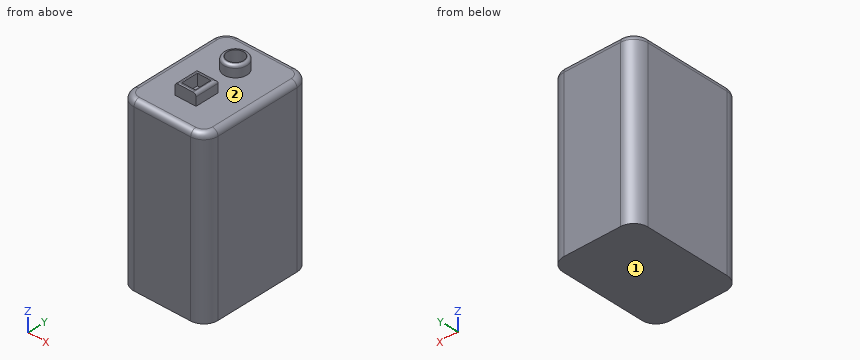
Autodesk Inventor part; units mm, degrees
ref_plane "YZ Plane" through (0, 0, 0) normal (1, 0, 0) x (0, 1, 0)
ref_plane "XZ Plane" through (0, 0, 0) normal (0, 1, 0) x (-1, 0, 0)
ref_plane "XY Plane" through (0, 0, 0) normal (0, 0, 1) x (1, 0, 0)
sketch "Sketch1" plane through (0, 0, 0) normal (1, 0, 0) x (0, 1, 0)
  line L0 (43.6864, 61.8662) -> (-7.1136, 61.8662)
  line L1 (-7.1136, 61.8662) -> (-7.1136, -14.3338)
  line L2 (-7.1136, -14.3338) -> (43.6864, -14.3338)
  line L3 (43.6864, -14.3338) -> (43.6864, 61.8662)
  point P0 (0, 0)
extrude "Extrusion1" add sketch "Sketch1" along normal blind 38.1
fillet "Fillet1" radius 6.35 4 edges at (38.1, 43.6864, 23.7662) (0, 43.6864, 23.7662) (38.1, -7.1136, 23.7662) (0, -7.1136, 23.7662)
sketch "Sketch2" plane through (0, -0.7636, 61.8662) normal (0, 0, 1) x (1, 0, 0)
  circle A0 centre (18.3636, 29.6461) radius 5.1979
  line L0 (14.0847, 15.7397) -> (23.5615, 15.7397)
  line L1 (23.5615, 15.7397) -> (23.5615, 5.0424)
  line L2 (23.5615, 5.0424) -> (14.0847, 5.0424)
  line L3 (14.0847, 5.0424) -> (14.0847, 15.7397)
  point P0 (0, 0.7636)
extrude "Extrusion2" add sketch "Sketch2" along normal blind 5.08
sketch "Sketch3" plane through (18.3636, 28.8825, 66.9462) normal (0, 0, 1) x (1, 0, 0)
  circle A0 centre (0, 0) radius 3.6755
  point P0 (-18.3636, -28.8825)
extrude "Extrusion3" cut sketch "Sketch3" against normal blind 5.08
sketch "Sketch4" plane through (0, -0.7636, 66.9462) normal (0, 0, 1) x (1, 0, 0)
  line L0 (15.8676, 13.9568) -> (21.9293, 13.9568)
  line L1 (21.9293, 13.9568) -> (21.9293, 7.1819)
  line L2 (21.9293, 7.1819) -> (15.8676, 7.1819)
  line L3 (15.8676, 7.1819) -> (15.8676, 13.9568)
  point P0 (0, 0.7636)
extrude "Extrusion4" cut sketch "Sketch4" against normal blind 5.08
fillet "Fillet2" radius 1.27 4 edges at (18.8231, 14.9761, 66.9462) (23.5615, 9.6275, 66.9462) (18.8984, 6.4183, 66.9462) (14.0847, 9.6275, 66.9462)
fillet "Fillet3" radius 1.27 1 edges at (13.1657, 28.8825, 66.9462)
fillet "Fillet4" radius 2.54 8 edges at (36.2401, 41.8266, 61.8662) (38.1, 18.2864, 61.8662) (36.2401, -5.2537, 61.8662) (19.05, -7.1136, 61.8662) (1.8599, -5.2537, 61.8662) (0, 18.2864, 61.8662) (1.8599, 41.8266, 61.8662) (19.05, 43.6864, 61.8662)
properties part number "Battery1" material "Lead"
The model under review builds one solid part; all positions refer to its coordinate system, in mm. Face numbers are marked on the shaded views. A direction names the side the tool comes from. Coordinates: 2 decimals unless noted, no trailing zeros. Write each loop counter-clockwise with the first axis right and the second up, starting at its lowest first coordinate (ties: lowest second). Pieces come first, ordered by that corner, then holes. Notation, with made-up numbers: (18.5, 7.25) - (68.5, 7.25) arc R25 ccw to (68.5, 21.25) - close; hole circle Ø2 at (69, -37.75). An arc over 180 degrees is marked (long way). Write item = value, one per line.
(1) Consider section B-B, the plane y = 9. Give the boundary of the cut face in (x, z), then the cut area to 3 significant figures.
Result sheet:
outline = (0, -14.33) - (38.1, -14.33) - (38.1, 59.33) arc R2.54 ccw to (35.56, 61.87) - (23.56, 61.87) - (23.56, 65.68) arc R1.27 ccw to (22.29, 66.95) - (21.93, 66.95) - (21.93, 61.87) - (15.87, 61.87) - (15.87, 66.95) - (15.35, 66.95) arc R1.27 ccw to (14.08, 65.68) - (14.08, 61.87) - (2.54, 61.87) arc R2.54 ccw to (0, 59.33) - close
area = 2,920 mm^2
(2) For line 1 (Z direction, x = 31.5, y = 3); line 2 (Y direction, x = 32, z = 16); line 3 (Z direction, x = 15.5, y = -5), list the stretches that pass through material, from the lowest coordinate up. Write a range as [from, to].
Result sheet:
line_1 = [-14.33, 61.87]
line_2 = [-7.11, 43.68]
line_3 = [-14.33, 61.83]
(3) Consider section C-C, the plane y = 2. Give the boundary of the cut face in (x, z).
Result sheet:
outline = (0, -14.33) - (38.1, -14.33) - (38.1, 59.33) arc R2.54 ccw to (35.56, 61.87) - (2.54, 61.87) arc R2.54 ccw to (0, 59.33) - close
(4) Machinability: for the marked faces 1 and 2, which of the approach directions +Z, -Z, +X, -X, +Y, -Y give a long, thin tool a straight path to every point of the face, cutting with its end or side? Answer none if there is none.
Result sheet:
face_1 = -Z, +X, -X, +Y, -Y
face_2 = +Z
(5) Consider section A-A, the plane z = 47. Give the boundary of the cut face in (x, y).
Result sheet:
outline = (0, -0.76) arc R6.35 ccw to (6.35, -7.11) - (31.75, -7.11) arc R6.35 ccw to (38.1, -0.76) - (38.1, 37.34) arc R6.35 ccw to (31.75, 43.69) - (6.35, 43.69) arc R6.35 ccw to (0, 37.34) - close
(6) For P1, Ø2.5, axis at x = 18, z = 65.5, coming from the -Y side; P2, Ø2.5, axis at y = 11, z = 65, coming from the -X side; P3, Ø2.5, axis at y = 9, z = 63.5, coming from the +X side, all flat-tipped, find the tip position at first contact; note any pin that passes through.
Result sheet:
P1 = 4.28
P2 = 14.08
P3 = 23.56
